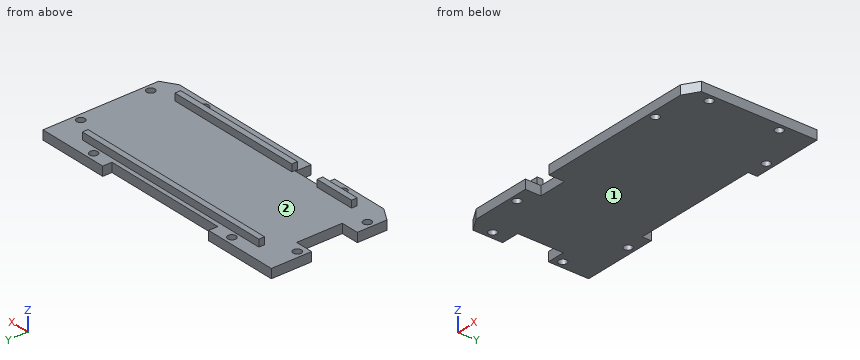
from build123d import *

# Parameters (mm, degrees)
TRIMMED_UPPER_SHELF_CABLE_NOTCH_AN_2_R       = 1.15
TRIMMED_UPPER_SHELF_CABLE_NOTCH_AND_AN_DEPTH = 2.6
PCB_START                                    = 2.6
PCB_EDGE_RESTS_WITH_ANTENNA_GAP_PROFILE_W    = 11.7
PCB_EDGE_RESTS_WITH_ANTENNA_GAP_PROFILE_H    = 1.6
PCB_EDGE_RESTS_WITH_ANTENNA_GAP_PROFILE_W_2  = 39.7
PCB_EDGE_RESTS_WITH_ANTENNA_GAP_PROFILE_W_3  = 60
PCB_EDGE_RESTS_WITH_ANTENNA_GAP_DEPTH        = 2


with BuildPart() as part:
    # Trimmed upper shelf - cable notch an 2 → Trimmed upper shelf - cable notch and an (new body)
    with BuildSketch(Plane.XY):
        Polygon((-38.8, -21.5), (-34.7, -24), (-18, -24), (-18, -19.6), (-10, -19.6), (-10, -24), (34.7, -24), (38.8, -21.5), (38.8, 11.2), (18.5, 11.2), (18.5, 8.6), (-17.5, 8.6), (-17.5, 11.2), (-38.8, 11.2), (-38.8, -0.2), (-33.7, -0.2), (-33.7, -13.1), (-38.8, -13.1), align=None)
        with Locations((-36.8, -17.6)):
            Circle(TRIMMED_UPPER_SHELF_CABLE_NOTCH_AN_2_R, mode=Mode.SUBTRACT)
        with Locations((36.8, -17.6)):
            Circle(TRIMMED_UPPER_SHELF_CABLE_NOTCH_AN_2_R, mode=Mode.SUBTRACT)
        with Locations((-36.8, 2.2)):
            Circle(TRIMMED_UPPER_SHELF_CABLE_NOTCH_AN_2_R, mode=Mode.SUBTRACT)
        with Locations((36.8, 2.2)):
            Circle(TRIMMED_UPPER_SHELF_CABLE_NOTCH_AN_2_R, mode=Mode.SUBTRACT)
        with Locations((-23, -22.2)):
            Circle(TRIMMED_UPPER_SHELF_CABLE_NOTCH_AN_2_R, mode=Mode.SUBTRACT)
        with Locations((24, -22.2)):
            Circle(TRIMMED_UPPER_SHELF_CABLE_NOTCH_AN_2_R, mode=Mode.SUBTRACT)
        with Locations((-23, 9.2)):
            Circle(TRIMMED_UPPER_SHELF_CABLE_NOTCH_AN_2_R, mode=Mode.SUBTRACT)
        with Locations((24, 9.2)):
            Circle(TRIMMED_UPPER_SHELF_CABLE_NOTCH_AN_2_R, mode=Mode.SUBTRACT)
    extrude(amount=TRIMMED_UPPER_SHELF_CABLE_NOTCH_AND_AN_DEPTH)

    # PCB edge rests with antenna gap profile → PCB edge rests with antenna gap (add)
    with BuildSketch(Plane.XY.offset(PCB_START)):
        with Locations((-24.15, -19.6)):
            Rectangle(PCB_EDGE_RESTS_WITH_ANTENNA_GAP_PROFILE_W, PCB_EDGE_RESTS_WITH_ANTENNA_GAP_PROFILE_H)
        with Locations((10.15, -19.6)):
            Rectangle(PCB_EDGE_RESTS_WITH_ANTENNA_GAP_PROFILE_W_2, PCB_EDGE_RESTS_WITH_ANTENNA_GAP_PROFILE_H)
        with Locations((0, 6.6)):
            Rectangle(PCB_EDGE_RESTS_WITH_ANTENNA_GAP_PROFILE_W_3, PCB_EDGE_RESTS_WITH_ANTENNA_GAP_PROFILE_H)
    extrude(amount=PCB_EDGE_RESTS_WITH_ANTENNA_GAP_DEPTH)


solid = part.part
For this review, take the finished solid that the model builds, in its own axes (mm). Face numbers are marked on the shaded views. Coordinates: 2 decimals unless noted, no trailing zeros. Write each loop counter-clockwise with the first axis right and the second up, starting at its lowest first coordinate (ties: lowest second). Pieces come first, ordered by that corner, then holes. Notation, with made-up numbers: (-34.75, -18.75) -> (-27.75, -18.75) arc R17 ccw to (-27.75, 8.25) -> close; hole circle Ø3 at (-12.5, 64.25). An arc over 180 degrees is marked (long way). Write each question's results on one line, items separated by ' | '. Start each with the question number.
1) Consider section A-A (z = 1.75). Give the number of separate pieces and of enclosed holes in the cut face, plus the area to 3 significant figures.
2) Consider section D-D (x = -15). Write out the cut boundary in (y, z), plus the area to 3 significant figures.
3) Insertion check: pin 1 (2 mm diameter, centred on x = 1, z = 3.5, fed in from -Y); pin 2 (2 mm diameter, centred on x = 7, y = -7, fed in from +Z); pin 3 (0.6 mm diameter, centred on x = -3.5, z = 4, fed in from -Y); pin 4 (2 mm diameter, centred on x = 24, y = -22.2, fed in from -Z). Each pin has a flat end and moves straight along its axis. Give the tip position at first contact, or say it passes through.
4) Consider section C-C (x = 24). Write out the cut boundary in (y, z).
5) Wall thickness on L1, parallel to X at y = -21.5, z = 0.45; L2, parallel to Z at x = 29, y = 3; L3, parallel to Y at x = -26, z = 3.15: over which ranges is each line inside the solid? List them lowest first. Write a range as [from, to].
6) The part is to be moulded in two halves that separate along Y. For the marked faces 1 and 2, say which applies: +Y half, -Y half, draft (parallel to the pull), parting line (faces both ways), or undercut.
7) Consider section B-B (y = -17.6). Write out the cut boundary in (x, z), plus the area to 3 significant figures.
Geometry says:
1) separate pieces: 1 | enclosed holes: 8 | area: 2,490 mm^2
2) outline: (-19.6, 0) -> (8.6, 0) -> (8.6, 2.6) -> (7.4, 2.6) -> (7.4, 4.6) -> (5.8, 4.6) -> (5.8, 2.6) -> (-19.6, 2.6) -> close | area: 76.5 mm^2
3) pin 1: y = -24 | pin 2: z = 2.6 | pin 3: y = -20.4 | pin 4: through
4) outline: (-24, 0) -> (-23.35, 0) -> (-23.35, 2.6) -> (-24, 2.6) -> close; (-21.05, 0) -> (8.05, 0) -> (8.05, 2.6) -> (7.4, 2.6) -> (7.4, 4.6) -> (5.8, 4.6) -> (5.8, 2.6) -> (-18.8, 2.6) -> (-18.8, 4.6) -> (-20.4, 4.6) -> (-20.4, 2.6) -> (-21.05, 2.6) -> close; (10.35, 0) -> (11.2, 0) -> (11.2, 2.6) -> (10.35, 2.6) -> close
5) L1: [-38.8, -23.91], [-22.09, -18], [-10, 23.09], [24.91, 38.8] | L2: [0, 2.6] | L3: [-20.4, -18.8], [5.8, 7.4]
6) face 1: draft | face 2: undercut
7) outline: (-38.8, 0) -> (-37.95, 0) -> (-37.95, 2.6) -> (-38.8, 2.6) -> close; (-35.65, 0) -> (35.65, 0) -> (35.65, 2.6) -> (-35.65, 2.6) -> close; (37.95, 0) -> (38.8, 0) -> (38.8, 2.6) -> (37.95, 2.6) -> close | area: 190 mm^2
